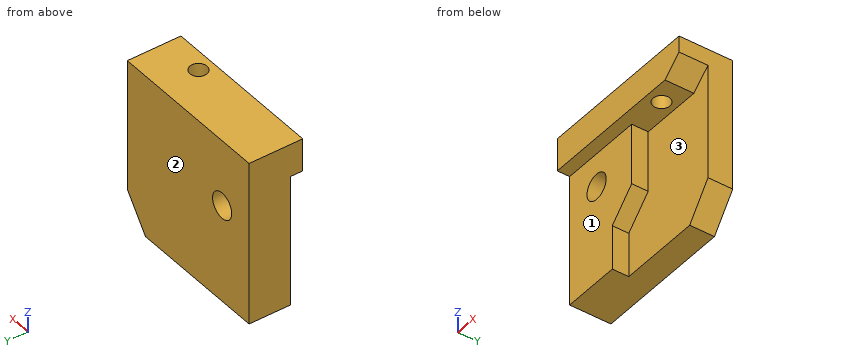
Autodesk Fusion 360 part; units mm, degrees
sketch "Sketch1" plane through (0, 0, 0) normal (0, 1, 0) x (1, 0, 0)
  line L0 (0, 0) -> (0, -200)
  line L1 (0, -200) -> (200, -200)
  line L2 (200, -200) -> (200, -40)
  line L3 (170, 0) -> (0, 0)
  line L4 (170, 0) -> (200, -40)
  line L5 (93.465, -147.4251) -> (198.1071, -147.4251)
  line L6 (93.465, -147.4251) -> (93.465, -145)
extrude "Extrude1" add sketch "Sketch1" along normal blind 30 makes body 1
sketch "Sketch2" plane through (0, 0, 0) normal (0, 1, 0) x (1, 0, 0)
  line L0 (0, -160) -> (197.6402, -160)
  line L1 (197.6402, -160) -> (200, -160)
  line L2 (101.8607, -160) -> (101.8607, -85.8975)
  line L3 (70, -53.971) -> (70, 0)
  line L4 (101.8607, -85.8975) -> (70, -53.971)
  line L5 (0, -160) -> (0, 0)
  line L6 (0, 0) -> (70, 0)
extrude "Extrude2" add sketch "Sketch2" against normal blind 20 separate body makes body 2
sketch "Sketch3" plane through (0, -20, 0) normal (0, -1, 0) x (1, 0, 0)
  line L0 (101.8607, 160) -> (0, 160)
  line L1 (0, 160) -> (0, 0)
  line L2 (0, 0) -> (70, 0)
  line L3 (70, 0) -> (70, 53.971)
  line L4 (70, 53.971) -> (101.8607, 85.8975)
  line L5 (101.8607, 85.8975) -> (101.8607, 160)
  line L6 (2.5338, 160) -> (176.8626, 160)
  line L7 (200, 160) -> (200, 200)
  line L8 (200, 200) -> (0, 200)
  line L9 (0, 200) -> (0, 160)
  line L10 (176.8626, 160) -> (200, 180)
extrude "Extrude3" add sketch "Sketch3" against normal blind 20 contours L0 L6 L7 L8 L9 L10 bodies 1 2
sketch "Sketch4" plane through (0, -20, 0) normal (0, -1, 0) x (1, 0, 0)
  line L0 (0, 200) -> (0, 0)
  line L1 (0, 0) -> (70, 0)
  line L2 (70, 0) -> (70, 53.971)
  line L3 (70, 53.971) -> (101.8607, 85.8975)
  line L4 (101.8607, 85.8975) -> (101.8607, 160)
  line L5 (101.8607, 160) -> (176.8626, 160)
  line L6 (176.8626, 160) -> (200, 180)
  line L7 (200, 180) -> (200, 200)
  line L8 (200, 200) -> (0, 200)
  line L9 (-5.5994, 160) -> (173.5818, 160)
  line L10 (200, 180) -> (200, 200)
  line L11 (0, 200) -> (0, 160)
extrude "Extrude4" add sketch "Sketch4" along normal blind 15 contours L0 L5 L6 L7 L8 L9 L10 L11 bodies 1
sketch "Sketch5" plane through (0, -20, 0) normal (0, -1, 0) x (1, 0, 0)
  line L0 (101.8607, 160) -> (0, 160)
  line L1 (0, 160) -> (0, 0)
  line L2 (0, 0) -> (70, 0)
  line L3 (70, 0) -> (70, 53.971)
  line L4 (70, 53.971) -> (101.8607, 85.8975)
  line L5 (101.8607, 85.8975) -> (101.8607, 160)
  circle A0 centre (44.2368, 119.0792) radius 15.737
extrude "Extrude5" cut sketch "Sketch5" against normal blind 60 contours A0 bodies 1
sketch "Sketch6" plane through (0, 0, 160) normal (0, 0, -1) x (1, 0, 0)
  line L0 (101.8607, 20) -> (101.8607, 0)
  line L1 (101.8607, 0) -> (176.8626, 0)
  line L2 (176.8626, 0) -> (176.8626, 35)
  line L3 (176.8626, 35) -> (0, 35)
  line L4 (0, 35) -> (0, 20)
  line L5 (0, 20) -> (101.8607, 20)
  circle A0 centre (147.113, 17.2318) radius 10.2876
extrude "Extrude6" cut sketch "Sketch6" against normal blind 40 contours A0 bodies 1
Work out the finished part from the listing and answer in its coordinate system (mm). Face numbers are marked on the shaded views. A direction names the side the tool comes from. Coordinates: 2 decimals unless noted, no trailing zeros. Write each loop counter-clockwise with the first axis right and the second up, starting at its lowest first coordinate (ties: lowest second). Pieces come first, ordered by that corner, then holes. Notation, with made-up numbers: M -20,36 L 16,36 A25 cw 16,67 Z; hole C 18.5,-2.5 d2. An arc over 180 degrees is marked long. Write item = value, one per line.
1. Flat-ended cylindrical pins translate along their axes: pin 1 (1.5 mm diameter, centred on y = -6, z = 29, fed in from +X); pin 2 (2 mm diameter, centred on x = 29, z = 132.5, fed in from -Y); pin 3 (16 mm diameter, centred on y = -12, z = 121, fed in from +X). Find the tip coordinate at first contact, or state that the pin passes through.
Solution:
pin_1 = 70
pin_2 = -20
pin_3 = 101.86
2. The part is cut by section B-B (x = 53.5). Determine the outline of the cut face in (y, z).
Solution:
outline = M -35,160 L -20,160 L -20,131.8 L 30,131.8 L 30,200 L -35,200 Z; M -20,0 L 30,0 L 30,106.36 L -20,106.36 Z
3. The part is cut by section D-D (x = 113). Determine the outline of the cut face in (y, z), then the cut area to 3 significant figures.
Solution:
outline = M -35,160 L 0,160 L 0,0 L 30,0 L 30,200 L -35,200 Z
area = 7,400 mm2
4. The part is cut by section A-A (y = -12.5). Determine the outline of the cut face in (x, z).
Solution:
outline = M 0,0 L 70,0 L 70,53.97 L 101.86,85.9 L 101.86,160 L 137.98,160 L 137.98,200 L 0,200 Z; M 156.25,160 L 176.86,160 L 200,180 L 200,200 L 156.25,200 Z; hole C 44.24,119.08 d31.47
5. The part is cut by section C-C (z = 128.5). Determine the outline of the cut face in (x, y).
Solution:
outline = M 0,-20 L 31.63,-20 L 31.63,30 L 0,30 Z; M 56.84,-20 L 101.86,-20 L 101.86,0 L 200,0 L 200,30 L 56.84,30 Z
6. Straight lines are drawn through the part: line 1 (X direction, y = -2, z = 96.5); line 2 (Y direction, x = 150, z = 150); line 3 (X direction, y = -7, z = 27.5). For each, find the intervals that lie inside material, in ascending order. Write a range as from..to.
Solution:
line_1 = 0..101.86
line_2 = 0..30
line_3 = 0..70
7. For the marked faces 1, 2 and 3, determine the directions among +Z, -Z, +X, -X, +Y, -Y from which every point of the face is accessible in a straight line to the end or side of a thin tool.
Solution:
face_1 = -Z, +X, -X, -Y
face_2 = +Z, -Z, +X, -X, +Y
face_3 = -Z, +X, -Y
